Build history of the part. All positions in model axes, mm. A direction names the side the tool comes from. Give positions to 0.01 mm unless a question says otherwise; leave off trailing zeros. Loops run counter-clockwise (first coordinate to the right, second up) from the corner with the lowest first, then second, coordinate; pieces in that order, holes last. Notation, with made-up numbers: (24, -36) - (61, -36) arc R24 ccw to (61, -7) - close; hole circle Ø4 at (85.25, -7). An arc over 180 degrees is marked (long way). Return JSON: item names as keys, results as strings. Group by question number.
1) Mould opens along X. For faces 1 (the face through (0.1, -1.9, 6.5)), 2 (the face through (-0.11, -1.93, -5.05)), 3 (the face through (6.2, -12.98, 1.95)) say: released by +X, released by -X, zero draft, split by the parting line, or undercut.
2) 3-axis set-ups, long thin cutter, end or side, ignore diameter. For faces 4 (the face through (4.817, -14.4, 1.517)), 5 (the face through (-0.846, 6.445, 0.301)): which of +Z, -Z, +X, -X, +Y, -Y reach the whole face in a straight line?
3) Drop flat-ended pins along their axis: pin 1 (3 mm diameter, centred on x = 1, z = -11.5, fed in from -Y); pin 2 (10 mm diameter, centred on y = -16, z = 7, fed in from -X); pin 3 (1.5 mm diameter, centred on x = 4, z = 3.5, fed in from -Y); pin 4 (3 mm diameter, centred on x = -2.5, z = 3.5, fed in from +Y). Give the stop position or say it passes through.
4) Slice it at A-A (y = -17.5). List the corners of the cut face in (x, z).
5) Drill centre line: probe 1 along X at (y, z) = (0, 8.5). Where is it in solid material? Low to high. Write a range as from..to.
```python
from build123d import *

# Parameters (mm, degrees)
F0_R     = 6.5
F0_R_2   = 5.05
F1_DEPTH = 25
F2_DEPTH = 25
F3_R     = 6.5
F3_R_2   = 5.05
F4_DEPTH = 25


# Not quite as in the source:
# - a fillet or chamfer that OpenCascade refuses, or shapes differently, is made with other operations: its cross-section is extruded or revolved along the edge and cut away or added


with BuildPart() as f1:
    # F0 (on Top) → F1 (new body)
    with BuildSketch(Plane.XY):
        Circle(F0_R)
        Circle(F0_R_2, mode=Mode.SUBTRACT)
    extrude(amount=F1_DEPTH)

    # F0 (on Top) → F2 (join)
    with BuildSketch(Plane.XY):
        Circle(F0_R)
        Circle(F0_R_2, mode=Mode.SUBTRACT)
    extrude(amount=-F2_DEPTH)

    # F3 (on Front) → F4 (join)
    with BuildSketch(Plane.XZ):
        Circle(F3_R)
        Circle(F3_R_2, mode=Mode.SUBTRACT)
    extrude(amount=F4_DEPTH)

    # F5: fillet of radius 5 on 3 edges, made by hand

    # F5_s1 → F5_t2 (revolve, cut)
    with BuildSketch(Plane.XY):
        with BuildLine():
            ThreePointArc((6.5, -21.4789916217), (6.1233105022, -23.3829348982), (5.05, -25))
            Line((5.05, -25), (6.5, -25))
            Line((6.5, -25), (6.5, -21.4789916217))
        make_face()
    revolve(axis=Axis((0, -25, 0), (0, -1, 0)), mode=Mode.SUBTRACT)

    # F5_s3 → F5_t4 (revolve, cut)
    with BuildSketch(Plane.XZ):
        with BuildLine():
            ThreePointArc((6.5, -21.4789916217), (6.1233105022, -23.3829348982), (5.05, -25))
            Line((5.05, -25), (6.5, -25))
            Line((6.5, -25), (6.5, -21.4789916217))
        make_face()
    revolve(axis=Axis((0, 0, -25), (0, 0, 1)), mode=Mode.SUBTRACT)

    # F5_s5 → F5_t6 (revolve, cut)
    with BuildSketch(Plane.XZ):
        with BuildLine():
            ThreePointArc((6.5, 21.4789916217), (6.1233105022, 23.3829348982), (5.05, 25))
            Line((5.05, 25), (6.5, 25))
            Line((6.5, 25), (6.5, 21.4789916217))
        make_face()
    revolve(axis=Axis((0, 0, 25), (0, 0, 1)), mode=Mode.SUBTRACT)


solid = f1.part
```
Results:
{
 "1": {"face 1": "undercut", "face 2": "undercut", "face 3": "split by the parting line"},
 "2": {"face 4": "-Y", "face 5": "none"},
 "3": {"pin 1": "y = -6.5", "pin 2": "x = -6.18", "pin 3": "y = -25", "pin 4": "y = 6.42"},
 "4": {"outline": "circle Ø13 at (0, 0); hole circle Ø10.1 at (0, 0)"},
 "5": {"probe 1": "-6.5..-5.05, 5.05..6.5"}
}
